from build123d import *

# Parameters (mm, degrees)
HOLES1_R           = 1.6
HOLES_DEPTH        = 3.5
HOLES_2_DEPTH      = 3.5
BOSS_EXTRUDE_DEPTH = 36
CUT_EXTRUDE1_DEPTH = 44.077981615
HOLE2_R            = 4.2
CUT_EXTRUDE2_DEPTH = 43.555992527


with BuildPart() as part:
    # Holes1 → Holes (new body)
    with BuildSketch(Plane(origin=(0, 0, 0), x_dir=(1, 0, 0), z_dir=(0, 1, 0))):
        with BuildLine():
            Line((-12.95, -3), (-7.95, -3))
            Line((-7.95, -3), (-7.95, 3))
            Line((-7.95, 3), (-12.95, 3))
            ThreePointArc((-12.95, 3), (-13.657106781, 2.707106781), (-13.95, 2))
            Line((-13.95, 2), (-13.95, -2))
            ThreePointArc((-13.95, -2), (-13.657106781, -2.707106781), (-12.95, -3))
        make_face()
        with Locations(Location((-11.2, 0, 0), (0, 0, 270))):
            Circle(HOLES1_R, mode=Mode.SUBTRACT)
    extrude(amount=HOLES_DEPTH)



with BuildPart() as body_2:
    # Holes1 → Holes 2 (new body)
    with BuildSketch(Plane(origin=(0, 0, 0), x_dir=(1, 0, 0), z_dir=(0, 1, 0))):
        with BuildLine():
            Line((7.95, 3), (7.95, -3))
            Line((7.95, -3), (12.95, -3))
            ThreePointArc((12.95, -3), (13.657106781, -2.707106781), (13.95, -2))
            Line((13.95, -2), (13.95, 2))
            ThreePointArc((13.95, 2), (13.657106781, 2.707106781), (12.95, 3))
            Line((12.95, 3), (7.95, 3))
        make_face()
        with Locations(Location((11.2, 0, 0), (0, 0, 270))):
            Circle(HOLES1_R, mode=Mode.SUBTRACT)
    extrude(amount=HOLES_2_DEPTH)


with BuildPart() as part_1:
    add(part.part)

    add(body_2.part)  # Boss-Extrude merges body 2
    # Sketch_3 → Boss-Extrude (add)
    with BuildSketch(Plane(origin=(0, 0, 0), x_dir=(1, 0, 0), z_dir=(0, 1, 0))):
        with BuildLine():
            Line((0, -8.95), (0, 8.95))
            Line((0, 8.95), (-6.95, 8.95))
            ThreePointArc((-6.95, 8.95), (-7.657106781, 8.657106781), (-7.95, 7.95))
            Line((-7.95, 7.95), (-7.95, 3))
            Line((-7.95, 3), (-7.95, -3))
            Line((-7.95, -3), (-7.95, -7.95))
            ThreePointArc((-7.95, -7.95), (-7.657106781, -8.657106781), (-6.95, -8.95))
            Line((-6.95, -8.95), (0, -8.95))
        make_face()
        with BuildLine():
            Line((6.95, 8.95), (0, 8.95))
            Line((0, 8.95), (0, -8.95))
            Line((0, -8.95), (6.95, -8.95))
            ThreePointArc((6.95, -8.95), (7.657106781, -8.657106781), (7.95, -7.95))
            Line((7.95, -7.95), (7.95, -3))
            Line((7.95, -3), (7.95, 3))
            Line((7.95, 3), (7.95, 7.95))
            ThreePointArc((7.95, 7.95), (7.657106781, 8.657106781), (6.95, 8.95))
        make_face()
    extrude(amount=BOSS_EXTRUDE_DEPTH)

    # CUT → Cut-Extrude1 (cut, through all)
    with BuildSketch(Plane.ZY.offset(7.95)):
        with BuildLine():
            Line((-4.25, 36), (4.25, 36))
            Line((4.25, 36), (4.25, 5))
            ThreePointArc((4.25, 5), (3.810660172, 3.939339828), (2.75, 3.5))
            Line((2.75, 3.5), (-2.75, 3.5))
            ThreePointArc((-2.75, 3.5), (-3.810660172, 3.939339828), (-4.25, 5))
            Line((-4.25, 5), (-4.25, 36))
        make_face()
    extrude(amount=-CUT_EXTRUDE1_DEPTH, mode=Mode.SUBTRACT)

    # Hole2 → Cut-Extrude2 (cut, through all)
    with BuildSketch(Plane.XY.offset(8.95)):
        with Locations((0, 28.05)):
            Circle(HOLE2_R)
        with BuildLine():
            Line((7.95, 36), (6.95, 36))
            Line((6.95, 36), (6.95, 31.910051813))
            ThreePointArc((6.95, 31.910051813), (7.695940488, 30.043740204), (7.95, 28.05))
            Line((7.95, 28.05), (7.95, 36))
        make_face()
        with BuildLine():
            Line((6.95, 36), (0, 36))
            ThreePointArc((0, 36), (4.032064489, 34.901638925), (6.95, 31.910051813))
            Line((6.95, 31.910051813), (6.95, 36))
        make_face()
        with BuildLine():
            Line((-6.95, 36), (-7.95, 36))
            Line((-7.95, 36), (-7.95, 28.05))
            ThreePointArc((-7.95, 28.05), (-7.695940488, 30.043740204), (-6.95, 31.910051813))
            Line((-6.95, 31.910051813), (-6.95, 36))
        make_face()
        with BuildLine():
            Line((0, 36), (-6.95, 36))
            Line((-6.95, 36), (-6.95, 31.910051813))
            ThreePointArc((-6.95, 31.910051813), (-4.032064489, 34.901638925), (0, 36))
        make_face()
    extrude(amount=-CUT_EXTRUDE2_DEPTH, mode=Mode.SUBTRACT)


solid = part_1.part
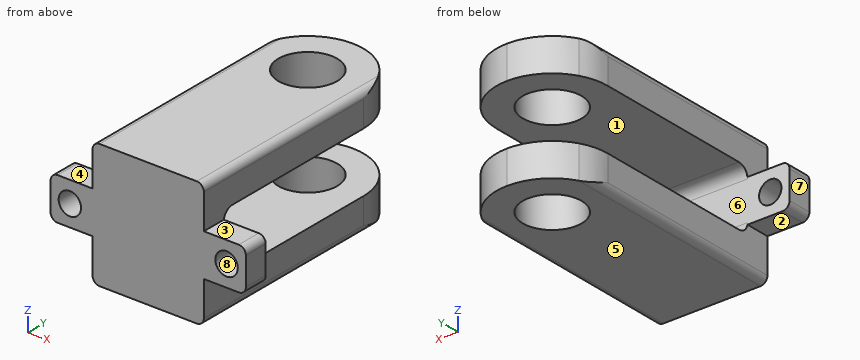
Can you work these out from the model? Positions are in its coordinate system, mm. Face numbers are marked on the shaded views. A direction names the side the tool comes from. Give positions to 0.01 mm unless a question says otherwise; leave off trailing zeros. Loops run counter-clockwise (first coordinate to the right, second up) from the corner with the lowest first, then second, coordinate; pieces in that order, holes last. Notation, with made-up numbers: M -39,-30.75 L -32,-30.75 A8 ccw -32,-20.75 Z; hole C 2.5,79 d2. An arc over 180 degrees is marked long. One line per item, written item: value.
1) I'm going to push flat-ended pins straight in: pin 1 (4 mm diameter, centred on x = 10, y = 1, fed in from +Z); pin 2 (5.5 mm diameter, centred on y = 8, z = 5, fed in from -X); pin 3 (1.8 mm diameter, centred on x = 9.5, y = 1.5, fed in from -Z). Where does each tip first touch, or does it pass through?
Geometry check:
pin 1: stops at z = 3
pin 2: stops at x = -7.95
pin 3: stops at z = -3
2) Imagine slicing it at D-D on y = 17. Write out the boundary of the cut face in (x, z), and give its area (3 significant figures).
Geometry check:
outline: M -7.95,-7.95 A1 ccw -6.95,-8.95 L 6.95,-8.95 A1 ccw 7.95,-7.95 L 7.95,-4.25 L -7.95,-4.25 Z; M -7.95,4.25 L 7.95,4.25 L 7.95,7.95 A1 ccw 6.95,8.95 L -6.95,8.95 A1 ccw -7.95,7.95 Z
area: 149 mm²
3) Imagine slicing it at C-C on y = 27. Write out the boundary of the cut face in (x, z).
Geometry check:
outline: M -7.95,-7.95 A1 ccw -6.95,-8.95 L -4.07,-8.95 L -4.07,-4.25 L -7.95,-4.25 Z; M -7.95,4.25 L -4.07,4.25 L -4.07,8.95 L -6.95,8.95 A1 ccw -7.95,7.95 Z; M 4.07,-8.95 L 6.95,-8.95 A1 ccw 7.95,-7.95 L 7.95,-4.25 L 4.07,-4.25 Z; M 4.07,4.25 L 7.95,4.25 L 7.95,7.95 A1 ccw 6.95,8.95 L 4.07,8.95 Z
4) Thinking about a two-plate mould opening in X: for the marked faces 6, 7 and 8, which applies, +X half, -X half, draft (parallel to the pull), parting line (faces both ways), or undercut?
Geometry check:
face 6: draft
face 7: -X half
face 8: undercut
5) On a 3-axis mill with a long thin cutter (end or side, diameter ignored), from which of +Z, -Z, +X, -X, +Y, -Y can I reach the whole of each face in a straight line? I mean the marked faces 1, 2, 3, 4 and 5. Say none if no direction works.
Geometry check:
face 1: +X, -X, +Y
face 2: -Z, -X, +Y, -Y
face 3: +Z, +X, +Y, -Y
face 4: +Z, -X, +Y, -Y
face 5: -Z, +X, -X, +Y, -Y
6) Imagine slicing it at B-B on x = 11.2. Write out the boundary of the cut face in (y, z).
Geometry check:
outline: M 0,-3 L 3.5,-3 L 3.5,-1.6 L 0,-1.6 Z; M 0,1.6 L 3.5,1.6 L 3.5,3 L 0,3 Z
7) Please list where these lines run through material, in increasing order: line 1 (X direction, y = 2.1, z = 0); line 2 (Z direction, x = 0.25, y = 10); line 3 (Y direction, x = -1.75, z = -1.75).
Geometry check:
line 1: x = -13.95 to -12.8, -9.6 to 9.6, 12.8 to 13.95
line 2: z = -8.95 to -4.25, 4.25 to 8.95
line 3: y = 0 to 3.5
8) Imagine slicing it at A-A on z = 0. Write out the boundary of the cut face in (x, y), and give its area (4 significant figures).
Geometry check:
outline: M -13.95,0 L -12.8,0 L -12.8,3.5 L -13.95,3.5 Z; M -9.6,0 L 9.6,0 L 9.6,3.5 L -9.6,3.5 Z; M 12.8,0 L 13.95,0 L 13.95,3.5 L 12.8,3.5 Z
area: 75.25 mm²
